```python
from build123d import *

# Parameters (mm, degrees)
F1_DEPTH = 9.525


with BuildPart() as f1:
    # F0 (on Front) → F1 (new body)
    with BuildSketch(Plane.XZ):
        with BuildLine():
            ThreePointArc((-19.547377, 34.395833), (-16.891, 22.225), (-19.547377, 10.054167))
            ThreePointArc((-19.547377, 10.054167), (-18.947889, 1.548851), (-11.465839, -2.54))
            Line((-11.465839, -2.54), (0, -2.54))
            Line((0, -2.54), (11.465839, -2.54))
            ThreePointArc((11.465839, -2.54), (18.947889, 1.548851), (19.547377, 10.054167))
            ThreePointArc((19.547377, 10.054167), (16.891, 22.225), (19.547377, 34.395833))
            ThreePointArc((19.547377, 34.395833), (18.947889, 42.901149), (11.465839, 46.99))
            Line((11.465839, 46.99), (0, 46.99))
            Line((0, 46.99), (-11.465839, 46.99))
            ThreePointArc((-11.465839, 46.99), (-18.947889, 42.901149), (-19.547377, 34.395833))
        make_face()
        with BuildLine():
            Line((11.465839, 0), (0, 0))
            Line((0, 0), (-11.465839, 0))
            ThreePointArc((-11.465839, 0), (-16.81016, 2.920608), (-17.238366, 8.995833))
            ThreePointArc((-17.238366, 8.995833), (-14.351, 22.225), (-17.238366, 35.454167))
            ThreePointArc((-17.238366, 35.454167), (-16.81016, 41.529392), (-11.465839, 44.45))
            Line((-11.465839, 44.45), (0, 44.45))
            Line((0, 44.45), (11.465839, 44.45))
            ThreePointArc((11.465839, 44.45), (16.81016, 41.529392), (17.238366, 35.454167))
            ThreePointArc((17.238366, 35.454167), (14.351, 22.225), (17.238366, 8.995833))
            ThreePointArc((17.238366, 8.995833), (16.81016, 2.920608), (11.465839, 0))
        make_face(mode=Mode.SUBTRACT)
    extrude(amount=F1_DEPTH)


solid = f1.part
```
Verification items for the finished model (mm, model axes). A direction names the side the tool comes from. Coordinates: 2 decimals unless noted, no trailing zeros. Loops run counter-clockwise (first coordinate to the right, second up) from the corner with the lowest first, then second, coordinate; pieces in that order, holes last. Notation, with made-up numbers: (57, 36) -> (109, 36) arc R11 ccw to (109, 52) -> close; hole circle Ø4 at (-39.5, -13.5). An arc over 180 degrees is marked (long way). Put each result on its own line as item: value.
1. Mould release check, pull along X, two halves, no side actions. Record for faces 1 (the face through (0, -5, 46.99)), 2 (the face through (19.01, -4.7, 42.8)), 3 (the face through (-18.88, -4.696, 43.005)), 4 (the face through (0, -5, 44.45)): pulls with the +X half, pulls with the -X half, needs draft (parallel to the pull), parting line crosses it, or undercut.
Result set:
face 1: needs draft
face 2: pulls with the +X half
face 3: pulls with the -X half
face 4: undercut
2. Section check A-A, the plane y = -8.5. Record the boundary of the cut face in (x, z) (3 decimals), then the cut area to 3 significant figures.
Result set:
outline: (-19.547, 10.054) arc R8.89 ccw to (-11.466, -2.54) -> (11.466, -2.54) arc R8.89 ccw to (19.547, 10.054) arc R29.21 cw to (19.547, 34.396) arc R8.89 ccw to (11.466, 46.99) -> (-11.466, 46.99) arc R8.89 ccw to (-19.547, 34.396) arc R29.21 cw to start; hole (-17.238, 8.996) arc R6.35 ccw to (-11.466, 0) -> (11.466, 0) arc R6.35 ccw to (17.238, 8.996) arc R31.75 cw to (17.238, 35.454) arc R6.35 ccw to (11.466, 44.45) -> (-11.466, 44.45) arc R6.35 ccw to (-17.238, 35.454) arc R31.75 cw to start
area: 404 mm^2
3. Tool access check on faces 5 (the face through (-16.762, -4.696, 2.846)), 6 (the face through (0, -5, -2.54)). Record the directions out of +Z, -Z, +X, -X, +Y, -Y that give a thin tool (end or side, any length) a straight path to the whole face; none if there is none.
Result set:
face 5: +Y, -Y
face 6: -Z, +X, -X, +Y, -Y
4. Section check C-C, the plane z = 31.5. Record the boundary of the cut face in (x, y) (3 decimals).
Result set:
outline: (-18.403, -9.525) -> (-15.736, -9.525) -> (-15.736, 0) -> (-18.403, 0) -> close; (15.736, -9.525) -> (18.403, -9.525) -> (18.403, 0) -> (15.736, 0) -> close
5. Thickness scan on line 1 (Z direction, x = 11, y = -7.5); line 2 (X direction, y = -5, z = 23); line 3 (Z direction, x = 13, y = -9). Record the ranges inside material, lowest first.
Result set:
line 1: z = -2.54 to 0, 44.45 to 46.99
line 2: x = -16.9 to -14.36, 14.36 to 16.9
line 3: z = -2.41 to 0.19, 44.26 to 46.86
6. Section check B-B, the plane x = 4. Record the boundary of the cut face in (y, z) (3 decimals), then the cut area to 3 significant figures.
Result set:
outline: (-9.525, -2.54) -> (0, -2.54) -> (0, 0) -> (-9.525, 0) -> close; (-9.525, 44.45) -> (0, 44.45) -> (0, 46.99) -> (-9.525, 46.99) -> close
area: 48.4 mm^2
7. Gauge pin test, flat ends, axial feed: P1, Ø1, axis at x = -13, y = -7.5, coming from the +Z side; P2, Ø1, axis at x = -15.5, y = -5.5, coming from the -Z side. Record the tip position at first contact, or that the pin passes through.
Result set:
P1: stops at z = 46.93
P2: stops at z = -1.81
